Could you check a few things on this model? Use its own coordinates, in mm. A direction names the side the tool comes from. Give positions to 0.01 mm unless a question says otherwise; leave off trailing zeros. Write each loop counter-clockwise with the first axis right and the second up, starting at its lowest first coordinate (ties: lowest second). Pieces come first, ordered by that corner, then holes. Notation, with made-up numbers: (53, 2) - (68, 2) arc R21 cw to (68, 38) - close; hole circle Ø7 at (36, 12). An arc over 180 degrees is marked (long way). Write item = value, one per line.
from build123d import *

# Parameters (mm, degrees)
SKETCH1_W           = 25.4
SKETCH1_H           = 50.8
SKETCH1_W_2         = 22.225
SKETCH1_H_2         = 47.625
EXTRUDE_THIN1_DEPTH = 508
SKETCH2_R           = 2.4765
CUT_EXTRUDE1_DEPTH  = 26.4
CUT_EXTRUDE2_REACH  = 52.8
SKETCH3_R           = 2.4892
CUT_EXTRUDE3_REACH  = 27.4
SKETCH4_R           = 3.175


with BuildPart() as part:
    # Sketch1 → Extrude-Thin1 (new body)
    with BuildSketch(Plane.XY):
        Rectangle(SKETCH1_W, SKETCH1_H)
        Rectangle(SKETCH1_W_2, SKETCH1_H_2, mode=Mode.SUBTRACT)
    extrude(amount=EXTRUDE_THIN1_DEPTH)

    # Sketch2 → Cut-Extrude1 (cut, through all)
    with BuildSketch(Plane(origin=(12.7, 0, 0), x_dir=(0, 0, -1), z_dir=(1, 0, 0))):
        with Locations((-457.2, 12.7)):
            Circle(SKETCH2_R)
        with Locations((-431.8, 12.7)):
            Circle(SKETCH2_R)
        with Locations((-431.8, -12.7)):
            Circle(SKETCH2_R)
        with Locations((-457.2, -12.7)):
            Circle(SKETCH2_R)
        with Locations((-165.1, 12.7)):
            Circle(SKETCH2_R)
        with Locations((-139.7, 12.7)):
            Circle(SKETCH2_R)
        with Locations((-139.7, -12.7)):
            Circle(SKETCH2_R)
        with Locations((-165.1, -12.7)):
            Circle(SKETCH2_R)
    extrude(amount=-CUT_EXTRUDE1_DEPTH, mode=Mode.SUBTRACT)

    # Sketch3 → Cut-Extrude2 (cut, up to next)
    with BuildSketch(Plane(origin=(0, 25.4, 0), x_dir=(1, 0, 0), z_dir=(0, 1, 0)), mode=Mode.PRIVATE) as cut_extrude2_sk1:
        with Locations((0, -323.85)):
            Circle(SKETCH3_R)
    cut_extrude2_tool1 = extrude(cut_extrude2_sk1.sketch, amount=-CUT_EXTRUDE2_REACH, mode=Mode.PRIVATE) & part.part
    add(cut_extrude2_tool1.solids().sort_by_distance((0, 25.4, 323.85))[0], mode=Mode.SUBTRACT)
    # Sketch3 → Cut-Extrude2 (cut, up to next)
    with BuildSketch(Plane(origin=(0, 25.4, 0), x_dir=(1, 0, 0), z_dir=(0, 1, 0)), mode=Mode.PRIVATE) as cut_extrude2_sk2:
        with Locations((0, -349.25)):
            Circle(SKETCH3_R)
    cut_extrude2_tool2 = extrude(cut_extrude2_sk2.sketch, amount=-CUT_EXTRUDE2_REACH, mode=Mode.PRIVATE) & part.part
    add(cut_extrude2_tool2.solids().sort_by_distance((0, 25.4, 349.25))[0], mode=Mode.SUBTRACT)
    # Sketch3 → Cut-Extrude2 (cut, up to next)
    with BuildSketch(Plane(origin=(0, 25.4, 0), x_dir=(1, 0, 0), z_dir=(0, 1, 0)), mode=Mode.PRIVATE) as cut_extrude2_sk3:
        with Locations((0, -476.25)):
            Circle(SKETCH3_R)
    cut_extrude2_tool3 = extrude(cut_extrude2_sk3.sketch, amount=-CUT_EXTRUDE2_REACH, mode=Mode.PRIVATE) & part.part
    add(cut_extrude2_tool3.solids().sort_by_distance((0, 25.4, 476.25))[0], mode=Mode.SUBTRACT)
    # Sketch3 → Cut-Extrude2 (cut, up to next)
    with BuildSketch(Plane(origin=(0, 25.4, 0), x_dir=(1, 0, 0), z_dir=(0, 1, 0)), mode=Mode.PRIVATE) as cut_extrude2_sk4:
        with Locations((0, -501.65)):
            Circle(SKETCH3_R)
    cut_extrude2_tool4 = extrude(cut_extrude2_sk4.sketch, amount=-CUT_EXTRUDE2_REACH, mode=Mode.PRIVATE) & part.part
    add(cut_extrude2_tool4.solids().sort_by_distance((0, 25.4, 501.65))[0], mode=Mode.SUBTRACT)

    # Sketch4 → Cut-Extrude3 (cut, up to next)
    with BuildSketch(Plane(origin=(12.7, 0, 0), x_dir=(0, 0, -1), z_dir=(1, 0, 0)), mode=Mode.PRIVATE) as cut_extrude3_sk1:
        with Locations((-25.4, 9.525)):
            Circle(SKETCH4_R)
    cut_extrude3_tool1 = extrude(cut_extrude3_sk1.sketch, amount=-CUT_EXTRUDE3_REACH, mode=Mode.PRIVATE) & part.part
    add(cut_extrude3_tool1.solids().sort_by_distance((12.7, 9.525, 25.4))[0], mode=Mode.SUBTRACT)
    # Sketch4 → Cut-Extrude3 (cut, up to next)
    with BuildSketch(Plane(origin=(12.7, 0, 0), x_dir=(0, 0, -1), z_dir=(1, 0, 0)), mode=Mode.PRIVATE) as cut_extrude3_sk2:
        with Locations((-6.35, 9.525)):
            Circle(SKETCH4_R)
    cut_extrude3_tool2 = extrude(cut_extrude3_sk2.sketch, amount=-CUT_EXTRUDE3_REACH, mode=Mode.PRIVATE) & part.part
    add(cut_extrude3_tool2.solids().sort_by_distance((12.7, 9.525, 6.35))[0], mode=Mode.SUBTRACT)
    # Sketch4 → Cut-Extrude3 (cut, up to next)
    with BuildSketch(Plane(origin=(12.7, 0, 0), x_dir=(0, 0, -1), z_dir=(1, 0, 0)), mode=Mode.PRIVATE) as cut_extrude3_sk3:
        with Locations((-6.35, -9.525)):
            Circle(SKETCH4_R)
    cut_extrude3_tool3 = extrude(cut_extrude3_sk3.sketch, amount=-CUT_EXTRUDE3_REACH, mode=Mode.PRIVATE) & part.part
    add(cut_extrude3_tool3.solids().sort_by_distance((12.7, -9.525, 6.35))[0], mode=Mode.SUBTRACT)
    # Sketch4 → Cut-Extrude3 (cut, up to next)
    with BuildSketch(Plane(origin=(12.7, 0, 0), x_dir=(0, 0, -1), z_dir=(1, 0, 0)), mode=Mode.PRIVATE) as cut_extrude3_sk4:
        with Locations((-25.4, -9.525)):
            Circle(SKETCH4_R)
    cut_extrude3_tool4 = extrude(cut_extrude3_sk4.sketch, amount=-CUT_EXTRUDE3_REACH, mode=Mode.PRIVATE) & part.part
    add(cut_extrude3_tool4.solids().sort_by_distance((12.7, -9.525, 25.4))[0], mode=Mode.SUBTRACT)


solid = part.part
1. If we section it at B-B, the plane y = -1: Please give me the cut outline in (x, z), and give its area (3 significant figures).
Filled sheet:
outline = (-12.7, 0) - (-11.11, 0) - (-11.11, 508) - (-12.7, 508) - close; (11.11, 0) - (12.7, 0) - (12.7, 508) - (11.11, 508) - close
area = 1,610 mm2
2. For pin 1 (4.5 mm diameter, centred on x = 0, z = 476.25, fed in from +Y); pin 2 (5.5 mm diameter, centred on y = -9.525, z = 25.4, fed in from +X), each with a flat end and sliding along its axis, tell me the tip position at first contact or that it passes through.
Filled sheet:
pin_1 = -23.81
pin_2 = -11.11
3. Which directions (+Z, -Z, +X, -X, +Y, -Y) give clear straight access to the entire face, cutting with the end or side of a thin tool? Please do faces 4 (the face through (0, -23.812, 250)), 5 (the face through (-11.3, 2, 508)).
Filled sheet:
face_4 = +Z, -Z
face_5 = +Z, +X, -X, +Y, -Y
4. If we section it at C-C, the plane z = 158: Please give me the cut outline in (x, y).
Filled sheet:
outline = (-12.7, -25.4) - (12.7, -25.4) - (12.7, 25.4) - (-12.7, 25.4) - close; hole (-11.11, -23.81) - (11.11, -23.81) - (11.11, 23.81) - (-11.11, 23.81) - close
5. Thinking about a two-plate mould opening in X: for faces 1 (the face through (-12.7, 0, 250)), 2 (the face through (11.112, 0, 250)), 3 (the face through (0, -25.4, 250)), which applies, pulls with the +X half, pulls with the -X half, needs draft (parallel to the pull), parting line crosses it, or undercut?
Filled sheet:
face_1 = pulls with the -X half
face_2 = undercut
face_3 = needs draft
6. If we section it at A-A, the plane x = 6.5: Please give me the cut outline in (y, z), and give its area (3 significant figures).
Filled sheet:
outline = (-25.4, 0) - (-23.81, 0) - (-23.81, 508) - (-25.4, 508) - close; (23.81, 0) - (25.4, 0) - (25.4, 508) - (23.81, 508) - close
area = 1,610 mm2
7. I need wall thicknesses on line 1 (Z direction, x = 0, y = 25); line 2 (X direction, y = 0.5, z = 407); line 3 (Y direction, x = -9, z = 237). Which ranges of each line are inside material? Lowest first, please.
Filled sheet:
line_1 = 0 to 321.36, 326.34 to 346.76, 351.74 to 473.76, 478.74 to 499.16, 504.14 to 508
line_2 = -12.7 to -11.11, 11.11 to 12.7
line_3 = -25.4 to -23.81, 23.81 to 25.4
